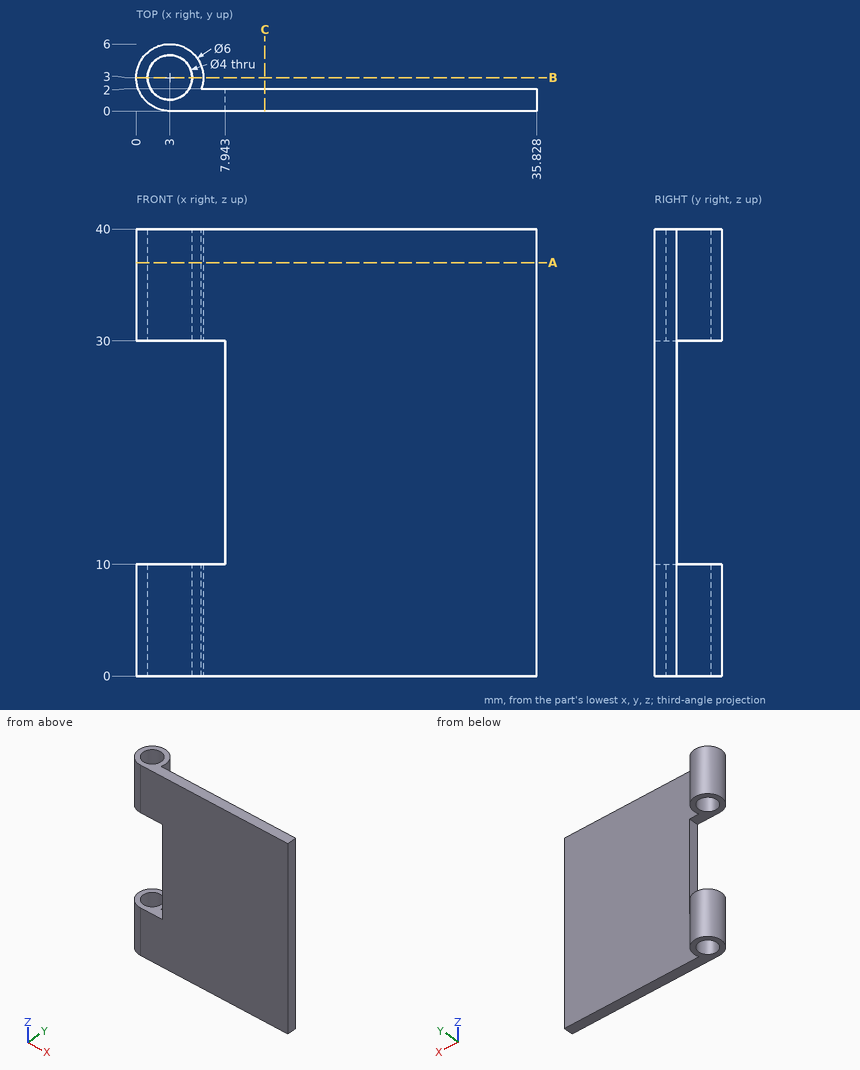
Check sheet for the drawn part. Datum: minimum x, y, z corner. Units: mm. Round coordinates to 2 decimals unless told otherwise and drop trailing zeros. Loops run counter-clockwise (first coordinate to the right, second up) from the corner with the lowest first, then second, coordinate; pieces in that order, holes last. Notation, with made-up numbers: (-19, 8) - (-7, 8) arc R19 ccw to (-7, 19) - close; hole circle Ø10 at (76.5, 22.5). An arc over 180 degrees is marked (long way). Write each question's results on one line, items separated by ' | '. Start each with the question number.
Q1. Cross-section at B-B on y = 3. Enter the section's corners in (x, z).
Q2. Cross-section at A-A on z = 37. Enter the section's corners in (x, y).
Q3. Thickness scan on line 1 (Y direction, x = 17.5, z = 12); line 2 (X direction, y = 1, z = 10.5); line 3 (X direction, y = 4, z = 30.5). Record the ranges inside material, lowest first. Write a range as [from, to].
Q4. Gauge pin test, flat ends, axial feed: P1, Ø6, axis at x = 29, z = 23.5, coming from the +Y side; P2, Ø3.5, axis at x = 3, y = 3, coming from the +Z side; P3, Ø3, axis at x = 5.5, y = 2.5, coming from the -Z side; P4, Ø0.6, axis at y = 1, z = 24, coming from the -X side. Record the tip position at first contact, or that the pin passes through.
Q5. Cross-section at C-C on x = 11.5. Enter the section's corners in (y, z).
Answers below:
1) outline: (0, 0) - (1, 0) - (1, 10) - (0, 10) - close; (0, 30) - (1, 30) - (1, 40) - (0, 40) - close; (5, 0) - (6, 0) - (6, 10) - (5, 10) - close; (5, 30) - (6, 30) - (6, 40) - (5, 40) - close
2) outline: (3, 0) - (35.83, 0) - (35.83, 2) - (5.83, 2) arc R3 ccw (long way) to start; hole circle Ø4 at (3, 3)
3) line 1: y = [0, 2] | line 2: x = [7.94, 35.83] | line 3: x = [0.17, 1.27], [4.73, 5.83]
4) P1: stops at y = 2 | P2: passes through | P3: stops at z = 0 | P4: stops at x = 7.94
5) outline: (0, 0) - (2, 0) - (2, 40) - (0, 40) - close
